Verification items for the finished model (mm, model axes). Face numbers are marked on the shaded views. A direction names the side the tool comes from. Round coordinates to 2 decimals unless told otherwise and drop trailing zeros. Loops run counter-clockwise (first coordinate to the right, second up) from the corner with the lowest first, then second, coordinate; pieces in that order, holes last. Notation, with made-up numbers: (-33.5, 79.5) -> (7.5, 79.5) arc R18 cw to (7.5, 112.5) -> close; hole circle Ø4 at (55.5, 64). An arc over 180 degrees is marked (long way). Use CSV: the item, a comma, the result in double quotes. Start each with the question number.
```python
from build123d import *

# Parameters (mm, degrees)
SKETCH_1_W                       = 50
SKETCH_1_H                       = 150
SM_BASE_FLANGE_1_DEPTH           = 2
SM_EDGE_FLANGE_1_STRIP_W         = 9.4732
SM_EDGE_FLANGE_1_STRIP_H         = 2
SM_EDGE_FLANGE_1_STRIP_CUT_DEPTH = 150
SM_EDGE_FLANGE_1_DEPTH           = 150
SKETCH_8_R                       = 3
CUT_EXTRUDE_1_DEPTH              = 10
PATTERN_LINEAR_1_COUNT           = 2
PATTERN_LINEAR_1_PITCH           = 100
FILLET_2_R                       = 5
FILLET_3_R                       = 5


# Sheet-metal steps are written as plain solids
with BuildPart() as part:
    # Sketch 1 → 基体-法兰1 (new body)
    with BuildSketch(Plane.XY):
        with Locations((16.662404092, -67.250639386)):
            Rectangle(SKETCH_1_W, SKETCH_1_H)
    extrude(amount=-SM_BASE_FLANGE_1_DEPTH)

    # 边线-法兰1 strip (across the edge) → 边线-法兰1 strip cut (cut)
    with BuildSketch(Plane(origin=(-8.337595908, 7.749360614, 0), x_dir=(1, 0, 0), z_dir=(0, -1, 0))):
        with Locations((-2, -1)):
            Rectangle(SM_EDGE_FLANGE_1_STRIP_W, SM_EDGE_FLANGE_1_STRIP_H)
    extrude(amount=SM_EDGE_FLANGE_1_STRIP_CUT_DEPTH, mode=Mode.SUBTRACT)

    # 边线-法兰1 section (across the edge) → 边线-法兰1 (add)
    with BuildSketch(Plane(origin=(-8.337595908, 7.749360614, 0), x_dir=(1, 0, 0), z_dir=(0, -1, 0))):
        with BuildLine():
            Line((0, 0.7366), (0, 128))
            Line((0, 128), (2, 128))
            Line((2, 128), (2, 0.7366))
            ThreePointArc((2, 0.7366), (2.215745145, 0.215745145), (2.7366, 0))
            Line((2.7366, 0), (2.7366, -2))
            ThreePointArc((2.7366, -2), (0.801531583, -1.198468417), (0, 0.7366))
        make_face()
    extrude(amount=SM_EDGE_FLANGE_1_DEPTH)

    # 草图8 → 切除-拉伸1 (cut)
    with BuildSketch(Plane.XY):
        with Locations((31.662404092, -22.250639386)):
            Circle(SKETCH_8_R)
    cut_extrude_1 = extrude(amount=-CUT_EXTRUDE_1_DEPTH, mode=Mode.SUBTRACT)

    # 阵列(线性)1: 切除-拉伸1 ×2
    with Locations(*[(0, -i * PATTERN_LINEAR_1_PITCH, 0) for i in range(1, PATTERN_LINEAR_1_COUNT)]):
        add(cut_extrude_1, mode=Mode.SUBTRACT)

    # 圆角2
    fillet_2_edges = [part.edges().sort_by_distance(p)[0] for p in [
        (-7.337595908, 7.749360614, 128),
    ]]
    fillet(fillet_2_edges, radius=FILLET_2_R)

    # 圆角3
    fillet_3_edges = [part.edges().sort_by_distance(p)[0] for p in [
        (-7.337595908, -142.250639386, 128),
    ]]
    fillet(fillet_3_edges, radius=FILLET_3_R)


solid = part.part
```
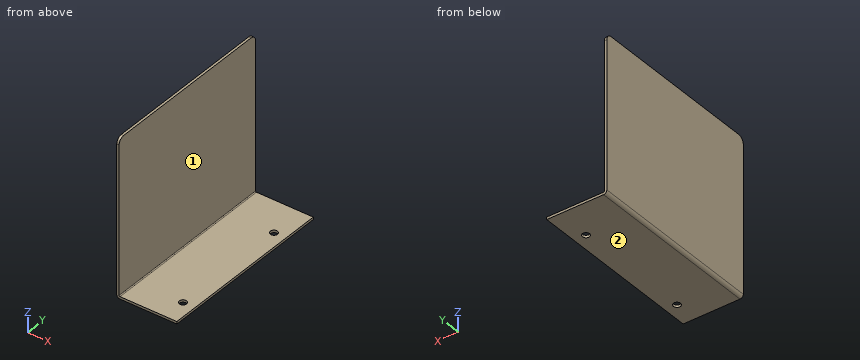
Q1. Thickness scan on L1, parallel to X at y = -11.5, z = 40; L2, parallel to Z at x = -1, y = -75.5. Record the ranges inside material, lowest first. Write a range as from..to.
Q2. Cross-section at C-C (z = 73.5). Record the boundary of the cut face in (x, y).
Q3. Cross-section at A-A (y = -104). Record the boundary of the cut face in (x, z).
Q4. Depth check by flat-ended pin: pin 1 Ø3.5 at (x, y) = (31.66, -122.25) entering from -Z; pin 2 Ø2 at (y, z) = (-101.5, 37) entering from +X. Enter the tip coordinate at first touch or a pass-through.
Q5. Cross-section at D-D (x = 6). Record the boundary of the cut face in (y, z).
Q6. Tool access check on the marked faces 1 and 2. Record the directions out of +Z, -Z, +X, -X, +Y, -Y that give a thin tool (end or side, any length) a straight path to the whole face; none if there is none.
Q7. Cross-section at B-B (x = 32). Record the boundary of the cut face in (y, z).
Answer list:
1,L1,"x = -8.34..-6.34"
1,L2,"z = -2..0"
2,outline,"(-8.34, -142.25) -> (-6.34, -142.25) -> (-6.34, 7.75) -> (-8.34, 7.75) -> close"
3,outline,"(-8.34, 0.74) arc R2.74 ccw to (-5.6, -2) -> (41.66, -2) -> (41.66, 0) -> (-5.6, 0) arc R0.74 cw to (-6.34, 0.74) -> (-6.34, 128) -> (-8.34, 128) -> close"
4,pin 1,"passes through"
4,pin 2,"stops at x = -6.34"
5,outline,"(-142.25, -2) -> (7.75, -2) -> (7.75, 0) -> (-142.25, 0) -> close"
6,face 1,"+Z, +X, +Y, -Y"
6,face 2,"-Z, +X, -X, +Y, -Y"
7,outline,"(-142.25, -2) -> (-125.23, -2) -> (-125.23, 0) -> (-142.25, 0) -> close; (-119.27, -2) -> (-25.23, -2) -> (-25.23, 0) -> (-119.27, 0) -> close; (-19.27, -2) -> (7.75, -2) -> (7.75, 0) -> (-19.27, 0) -> close"
